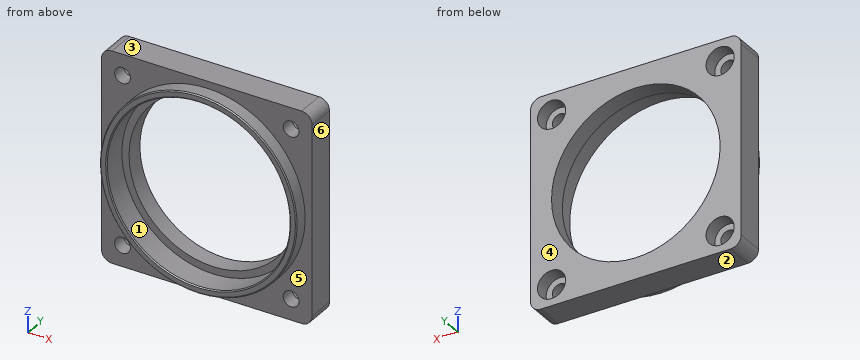
```python
from build123d import *

# Parameters (mm, degrees)
SKETCH_1_W          = 60
SKETCH_1_H          = 60
SKETCH_1_R          = 24
EXTRUDE_1_DEPTH     = 8
SKETCH_2_R          = 28
SKETCH_2_R_2        = 26
EXTRUDE_2_DEPTH     = 4
SKETCH_3_R          = 2.25
CUT_EXTRUDE_1_DEPTH = 44.17406629
FILLET_1_R          = 3
SKETCH_4_R          = 26.05
CUT_EXTRUDE_2_DEPTH = 7
SKETCH_5_R          = 4
CUT_EXTRUDE_3_DEPTH = 4
CHAMFER_1_SIZE      = 0.3


with BuildPart() as part:
    # Эскиз1 → Бобышка-Вытянуть1 (new body)
    with BuildSketch(Plane(origin=(0, 0, 0), x_dir=(1, 0, 0), z_dir=(0, 1, 0))):
        Rectangle(SKETCH_1_W, SKETCH_1_H)
        with Locations(Location((0, 0, 0), (0, 0, 270))):
            Circle(SKETCH_1_R, mode=Mode.SUBTRACT)
    extrude(amount=EXTRUDE_1_DEPTH)

    # Эскиз2 → Бобышка-Вытянуть2 (add)
    with BuildSketch(Plane.XZ):
        with Locations(Location((0, 0, 0), (0, 0, 270))):
            Circle(SKETCH_2_R)
        with Locations(Location((0, 0, 0), (0, 0, 270))):
            Circle(SKETCH_2_R_2, mode=Mode.SUBTRACT)
    extrude(amount=EXTRUDE_2_DEPTH)

    # Эскиз3 → Вырез-Вытянуть1 (cut, through all)
    with BuildSketch(Plane(origin=(0, 0, 0), x_dir=(-1, 0, 0), z_dir=(0, -1, 0))):
        with Locations(Location((24, -24, 0), (0, 0, 90))):
            Circle(SKETCH_3_R)
        with Locations(Location((-24, -24, 0), (0, 0, 90))):
            Circle(SKETCH_3_R)
        with Locations(Location((-24, 24, 0), (0, 0, 90))):
            Circle(SKETCH_3_R)
        with Locations(Location((24, 24, 0), (0, 0, 90))):
            Circle(SKETCH_3_R)
    extrude(amount=-CUT_EXTRUDE_1_DEPTH, mode=Mode.SUBTRACT)

    # Скругление1
    fillet_1_edges = [part.edges().sort_by_distance(p)[0] for p in [
        (30, 4, 30),
        (-30, 4, 30),
        (-30, 4, -30),
        (30, 4, -30),
    ]]
    fillet(fillet_1_edges, radius=FILLET_1_R)

    # Эскиз4 → Вырез-Вытянуть2 (cut)
    with BuildSketch(Plane.XZ.offset(4)):
        with Locations(Location((0, 0, 0), (0, 0, 270))):
            Circle(SKETCH_4_R)
    extrude(amount=-CUT_EXTRUDE_2_DEPTH, mode=Mode.SUBTRACT)

    # Эскиз5 → Вырез-Вытянуть3 (cut)
    with BuildSketch(Plane(origin=(0, 8, 0), x_dir=(1, 0, 0), z_dir=(0, 1, 0))):
        with Locations(Location((-24, 24, 0), (0, 0, 270))):
            Circle(SKETCH_5_R)
        with Locations(Location((24, 24, 0), (0, 0, 270))):
            Circle(SKETCH_5_R)
        with Locations(Location((24, -24, 0), (0, 0, 270))):
            Circle(SKETCH_5_R)
        with Locations(Location((-24, -24, 0), (0, 0, 270))):
            Circle(SKETCH_5_R)
    extrude(amount=-CUT_EXTRUDE_3_DEPTH, mode=Mode.SUBTRACT)

    # Фаска1
    chamfer_1_edges = [part.edges().sort_by_distance(p)[0] for p in [
        (0, -4, 28),
        (0, -4, 26.05),
    ]]
    chamfer(chamfer_1_edges, length=CHAMFER_1_SIZE)


solid = part.part
```
The model under review builds one solid part; all positions refer to its coordinate system, in mm. Face numbers are marked on the shaded views. A direction names the side the tool comes from. Round coordinates to 2 decimals unless told otherwise and drop trailing zeros. Order: outer loops, then holes, each group sorted by start corner. A loop starts at its lowest first (then second) coordinate and runs counter-clockwise, first axis right, second up.
Item 1: To check wall thickness, follow probe 1 along X at (y, z) = (5.5, 21.5); probe 2 along X at (y, z) = (2.75, 24); probe 3 along X at (y, z) = (1.75, 0). State the ranges of each line that lie inside material, in increasing order.
Working result:
probe 1: x = -30 to -27.12, -20.88 to -10.67, 10.67 to 20.88, 27.12 to 30
probe 2: x = -30 to -26.25, -21.75 to -10.13, 10.13 to 21.75, 26.25 to 30
probe 3: x = -30 to -26.05, 26.05 to 30
Item 2: Draft analysis for pull direction Z (two halves, no side actions). For the marked faces 1, 2, 3 and 4, state which applies: released by +Z, released by -Z, zero draft, split by the parting line, or undercut.
Working result:
face 1: undercut
face 2: released by -Z
face 3: released by +Z
face 4: zero draft
Item 3: Machinability: for the marked faces 5 and 6, which of the approach directions +Z, -Z, +X, -X, +Y, -Y give a long, thin tool a straight path to every point of the face, cutting with its end or side? Answer none if there is none.
Working result:
face 5: -Y
face 6: +Z, -Z, +X, +Y, -Y
Item 4: Add section C-C, the plane y = 5.25. State the section outline as (x, z) points, and give its area (3 significant figures).
Working result:
outline: (-30, -27) arc R3 ccw to (-27, -30) - (27, -30) arc R3 ccw to (30, -27) - (30, 27) arc R3 ccw to (27, 30) - (-27, 30) arc R3 ccw to (-30, 27) - close; hole circle Ø8 at (-24, -24); hole circle Ø8 at (-24, 24); hole circle Ø48 at (0, 0); hole circle Ø8 at (24, -24); hole circle Ø8 at (24, 24)
area: 1,580 mm2
Item 5: Add section A-A, the plane z = 0. State the section outline as (x, y) points.
Working result:
outline: (-30, 0) - (-28, 0) - (-28, -3.7) - (-27.7, -4) - (-26.35, -4) - (-26.05, -3.7) - (-26.05, 3) - (-24, 3) - (-24, 8) - (-30, 8) - close; (24, 3) - (26.05, 3) - (26.05, -3.7) - (26.35, -4) - (27.7, -4) - (28, -3.7) - (28, 0) - (30, 0) - (30, 8) - (24, 8) - close
Item 6: For pin 1 (18 mm diameter, centred on x = -5.5, z = 13.5, fed in from -Y); pin 2 (10.5 mm diameter, centred on x = 24, z = -24, fed in from -Y); pin 3 (5 mm diameter, centred on x = 24, z = 24, fed in from +Y), all flat-tipped, find the tip position at first contact; note any pin that passes through.
Working result:
pin 1: passes through
pin 2: stops at y = 0
pin 3: stops at y = 4
Item 7: Add section B-B, the plane x = 0. State the section outline as (y, z) points.
Working result:
outline: (-4, -27.7) - (-3.7, -28) - (0, -28) - (0, -30) - (8, -30) - (8, -24) - (3, -24) - (3, -26.05) - (-3.7, -26.05) - (-4, -26.35) - close; (-4, 26.35) - (-3.7, 26.05) - (3, 26.05) - (3, 24) - (8, 24) - (8, 30) - (0, 30) - (0, 28) - (-3.7, 28) - (-4, 27.7) - close
